from build123d import *

# Parameters (mm, degrees)
PAD_DEPTH = 15


with BuildPart() as part:
    # Sketch → Pad (new body)
    with BuildSketch(Plane.XY):
        Polygon((0, 30), (30.417592, 63.162781), (23.454944, 18.704694), (68.34771, 15.599919), (29.247837, -6.675628), (54.810608, -43.710001), (13.016512, -27.029066), (0, -70.105398), (-13.016512, -27.029066), (-54.810608, -43.710001), (-29.247837, -6.675628), (-68.34771, 15.599919), (-23.454944, 18.704694), (-30.417592, 63.162781), align=None)
    extrude(amount=PAD_DEPTH)

    # Sketch001 → Groove (revolve, cut)
    with BuildSketch(Plane.XZ):
        Polygon((0, 90.473419), (0, 14.138247), (80.88575, 2.052736), (80.88575, 90.473419), align=None)
    revolve(axis=Axis((0, 0, 0), (0, 0, 1)), mode=Mode.SUBTRACT)


solid = part.part
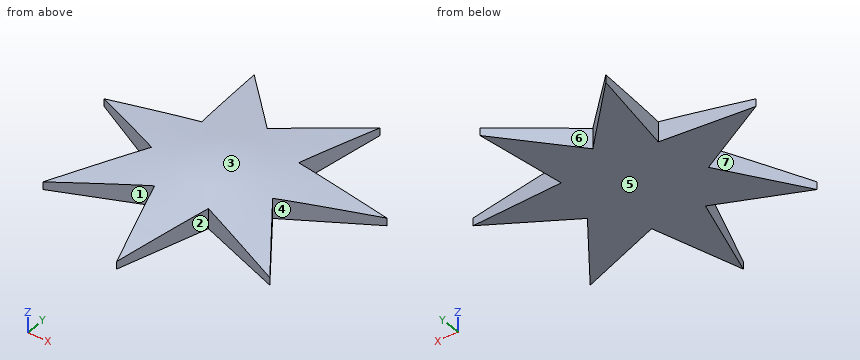
For this review, take the finished solid that the model builds, in its own axes (mm). Face numbers are marked on the shaded views. A direction names the side the tool comes from. Coordinates: 2 decimals unless noted, no trailing zeros. Return JSON: item names as keys, results as strings.
1. The part is to be moulded in two halves that separate along X. For the marked faces 1, 2, 3 and 4, say which applies: +X half, -X half, draft (parallel to the pull), parting line (faces both ways), or undercut.
Answer block:
{"face 1": "undercut", "face 2": "undercut", "face 3": "parting line", "face 4": "+X half"}
2. For line 1 (Y direction, x = 35.5, z = 3.75); line 2 (Y direction, x = 34, z = 2.5); line 3 (X direction, y = -52.5, z = 2), list the stretches that pass through material, from the lowest coordinate up. Write a range as from..to.
Answer block:
{"line 1": "-36..-15.73, -3.11..17.87", "line 2": "-35.4..-13.56, -3.97..17.98", "line 3": "-5.32..5.32"}
3. For pin 1 Ø8 at (x, y) = (-37.5, -25) entering from +Z; pin 2 Ø1 at (x, z) = (-35.5, 5) entering from +Y; pin 3 Ø1 at (y, z) = (-21, 7) entering from +X, all flat-tipped, find the tip position at first contact; note any pin that passes through.
Answer block:
{"pin 1": "z = 8", "pin 2": "y = 17.91", "pin 3": "x = 39.48"}
4. Machinability: for the marked faces 5, 6 and 7, which of the approach directions +Z, -Z, +X, -X, +Y, -Y give a long, thin tool a straight path to every point of the face, cutting with its end or side? Answer none if there is none.
Answer block:
{"face 5": "-Z, +X, -X, +Y, -Y", "face 6": "+Z, -Z, +Y", "face 7": "+Z, -Z, -X"}
